Check sheet for the modelled part. Datum: model origin and axes. Units: mm. A direction names the side the tool comes from. Give positions to 0.01 mm unless a question says otherwise; leave off trailing zeros. Order: outer loops, then holes, each group sorted by start corner. A loop starts at its lowest first (then second) coordinate and runs counter-clockwise, first axis right, second up. Notation, with made-up numbers: (69.25, 23) -> (74.25, 23) arc R35 cw to (74.25, 55) -> close; hole circle Ø8 at (0.25, -22.5). An arc over 180 degrees is marked (long way). Answer in a Markdown table with one row per item. Add a question column.
(1) Set-up check for faces 4 (the face through (87, 3, -105)), 5 (the face through (20, 3, -102)), 6 (the face through (55, 3, -20.322)), 7 (the face through (20, 3, -40)): record each of +Z, -Z, +X, -X, +Y, -Y from which the full face is reachable in a straight line by a thin tool's end or side.
(2) Cross-section at A-A (x = 62.5). Record the cut outline in (y, z).
(3) Cross-section at B-B (z = -17). Record the cut outline in (x, y).
(4) Release check for a two-part mould opening along X. For faces 1 (the face through (97, 3, -105)), 2 (the face through (35, 3, -47)), 3 (the face through (29.574, 3.042, -82.14)) record: released by +X, released by -X, zero draft, split by the parting line, or undercut.
(5) Thickness scan on L1, parallel to X at y = 3, z = -48; L2, parallel to X at y = 2.75, z = -44; L3, parallel to X at y = 1.85, z = -17. Record the ranges inside material, lowest first. Write a range as [from, to].
(6) Go/stop test with flat-tipped pins: pin 1 (8.5 mm diameter, centred on x = 70, z = -8, fed in from +Y); pin 2 (2.5 mm diameter, centred on y = 2.5, z = -18.5, fed in from -X); pin 3 (1.4 mm diameter, centred on x = 51.5, y = 2.5, fed in from -Z); pin 4 (3 mm diameter, centred on x = 85, z = -8, fed in from +Y). Record where each tip stops, or that it passes through.
```python
from build123d import *

# Parameters (mm, degrees)
SKETCH1_W           = 100
SKETCH1_H           = 105
BOSS_EXTRUDE1_DEPTH = 6
SKETCH3_W           = 10
SKETCH3_H           = 5
SKETCH3_W_2         = 15
SKETCH3_W_3         = 20
SKETCH3_W_4         = 25
SKETCH3_W_5         = 30
SKETCH3_W_6         = 35
SKETCH3_W_7         = 40
SKETCH3_W_8         = 45
SKETCH3_W_9         = 50
SKETCH3_W_10        = 55
CUT_EXTRUDE1_DEPTH  = 6
SKETCH4_W           = 5
SKETCH4_H           = 80
SKETCH4_H_2         = 75
SKETCH4_H_3         = 70
SKETCH4_H_4         = 65
SKETCH4_H_5         = 60
CUT_EXTRUDE2_DEPTH  = 6
SKETCH5_R           = 1.35
SKETCH5_R_2         = 1.6
SKETCH5_R_3         = 2.1
SKETCH5_R_4         = 2.6
SKETCH5_R_5         = 1.1
SKETCH5_R_6         = 3.1
SKETCH5_R_7         = 3.6
SKETCH5_R_8         = 4.1
CUT_EXTRUDE3_DEPTH  = 7
SKETCH7_W           = 5
SKETCH7_H           = 5
SKETCH7_H_2         = 6
SKETCH7_H_3         = 8
CUT_EXTRUDE4_DEPTH  = 7
CUT_EXTRUDE5_DEPTH  = 7


with BuildPart() as part:
    # Sketch1 → Boss-Extrude1 (new body)
    with BuildSketch(Plane(origin=(0, 0, 0), x_dir=(1, 0, 0), z_dir=(0, 1, 0))):
        with Locations((50, 52.5)):
            Rectangle(SKETCH1_W, SKETCH1_H)
    extrude(amount=BOSS_EXTRUDE1_DEPTH)

    # Sketch3 → Cut-Extrude1 (cut)
    with BuildSketch(Plane(origin=(0, 6, 0), x_dir=(1, 0, 0), z_dir=(0, 1, 0))):
        with Locations((5, 97.5)):
            Rectangle(SKETCH3_W, SKETCH3_H)
        with Locations((7.5, 87.5)):
            Rectangle(SKETCH3_W_2, SKETCH3_H)
        with Locations((10, 77.5)):
            Rectangle(SKETCH3_W_3, SKETCH3_H)
        with Locations((12.5, 67.5)):
            Rectangle(SKETCH3_W_4, SKETCH3_H)
        with Locations((15, 57.5)):
            Rectangle(SKETCH3_W_5, SKETCH3_H)
        with Locations((17.5, 47.5)):
            Rectangle(SKETCH3_W_6, SKETCH3_H)
        with Locations((20, 37.5)):
            Rectangle(SKETCH3_W_7, SKETCH3_H)
        with Locations((22.5, 27.5)):
            Rectangle(SKETCH3_W_8, SKETCH3_H)
        with Locations((25, 17.5)):
            Rectangle(SKETCH3_W_9, SKETCH3_H)
        with Locations((27.5, 7.5)):
            Rectangle(SKETCH3_W_10, SKETCH3_H)
    extrude(amount=-CUT_EXTRUDE1_DEPTH, mode=Mode.SUBTRACT)

    # Sketch4 → Cut-Extrude2 (cut)
    with BuildSketch(Plane(origin=(0, 6, 0), x_dir=(1, 0, 0), z_dir=(0, 1, 0))):
        with Locations((92.5, 65)):
            Rectangle(SKETCH4_W, SKETCH4_H)
        with Locations((82.5, 67.5)):
            Rectangle(SKETCH4_W, SKETCH4_H_2)
        with Locations((72.5, 70)):
            Rectangle(SKETCH4_W, SKETCH4_H_3)
        with Locations((62.5, 72.5)):
            Rectangle(SKETCH4_W, SKETCH4_H_4)
        with Locations((52.5, 75)):
            Rectangle(SKETCH4_W, SKETCH4_H_5)
    extrude(amount=-CUT_EXTRUDE2_DEPTH, mode=Mode.SUBTRACT)

    # Sketch5 → Cut-Extrude3 (cut, through all)
    with BuildSketch(Plane(origin=(0, 6, 0), x_dir=(1, 0, 0), z_dir=(0, 1, 0))):
        with Locations((91, 8)):
            Circle(SKETCH5_R)
        with Locations((85, 8)):
            Circle(SKETCH5_R_2)
        with Locations((78, 8)):
            Circle(SKETCH5_R_3)
        with Locations((70, 8)):
            Circle(SKETCH5_R_4)
        with Locations((96, 8)):
            Circle(SKETCH5_R_5)
        with Locations((90, 17)):
            Circle(SKETCH5_R_6)
        with Locations((80, 17)):
            Circle(SKETCH5_R_7)
        with Locations((69, 17)):
            Circle(SKETCH5_R_8)
    extrude(amount=-CUT_EXTRUDE3_DEPTH, mode=Mode.SUBTRACT)

    # Sketch7 → Cut-Extrude4 (cut, through all)
    with BuildSketch(Plane(origin=(0, 6, 0), x_dir=(1, 0, 0), z_dir=(0, 1, 0))):
        with Locations((22.5, 102.5)):
            Rectangle(SKETCH7_W, SKETCH7_H)
        with Locations((32.5, 102)):
            Rectangle(SKETCH7_W, SKETCH7_H_2)
        with Locations((42.5, 101)):
            Rectangle(SKETCH7_W, SKETCH7_H_3)
    extrude(amount=-CUT_EXTRUDE4_DEPTH, mode=Mode.SUBTRACT)

    # Sketch8 → Cut-Extrude5 (cut, through all)
    with BuildSketch(Plane(origin=(0, 6, 0), x_dir=(1, 0, 0), z_dir=(0, 1, 0))):
        Polygon((65.986104675, 31.416856683), (64.340656408, 34.266856683), (61.049759874, 34.266856683), (59.404311607, 31.416856683), (61.049759874, 28.566856683), (64.340656408, 28.566856683), align=None)
        Polygon((59.309574734, 23.921668245), (57.231113764, 27.521668245), (53.074191826, 27.521668245), (50.995730857, 23.921668245), (53.074191826, 20.321668245), (57.231113764, 20.321668245), align=None)
        Polygon((55.845473118, 34.972078883), (53.478337015, 39.072078883), (48.744064807, 39.072078883), (46.376928704, 34.972078883), (48.744064807, 30.872078883), (53.478337015, 30.872078883), align=None)
        Polygon((46.037567534, 60.151166507), (43.093081161, 65.251166507), (37.204108416, 65.251166507), (34.259622043, 60.151166507), (37.204108416, 55.051166507), (43.093081161, 55.051166507), align=None)
        Polygon((42.884078391, 78.793578101), (39.073566615, 85.393578101), (31.452543062, 85.393578101), (27.642031285, 78.793578101), (31.452543062, 72.193578101), (39.073566615, 72.193578101), align=None)
    extrude(amount=-CUT_EXTRUDE5_DEPTH, mode=Mode.SUBTRACT)


solid = part.part
```
Answer below:
| question | item | result |
|---|---|---|
| 1 | face 4 | -Z, +X, -X, +Y, -Y |
| 1 | face 5 | -Z, +Y, -Y |
| 1 | face 6 | +Y, -Y |
| 1 | face 7 | -X, +Y, -Y |
| 2 | outline | (0, -40) -> (6, -40) -> (6, -34.27) -> (0, -34.27) -> close; (0, -28.57) -> (6, -28.57) -> (6, 0) -> (0, 0) -> close |
| 3 | outline | (50, 0) -> (64.9, 0) -> (64.9, 6) -> (50, 6) -> close; (73.1, 0) -> (76.4, 0) -> (76.4, 6) -> (73.1, 6) -> close; (83.6, 0) -> (86.9, 0) -> (86.9, 6) -> (83.6, 6) -> close; (93.1, 0) -> (100, 0) -> (100, 6) -> (93.1, 6) -> close |
| 4 | face 1 | zero draft |
| 4 | face 2 | released by -X |
| 4 | face 3 | undercut |
| 5 | L1 | x = [35, 50], [55, 60], [65, 70], [75, 80], [85, 90], [95, 100] |
| 5 | L2 | x = [0, 60], [65, 70], [75, 80], [85, 90], [95, 100] |
| 5 | L3 | x = [50, 64.9], [73.1, 76.4], [83.6, 86.9], [93.1, 100] |
| 6 | pin 1 | stops at y = 6 |
| 6 | pin 2 | stops at x = 50 |
| 6 | pin 3 | stops at z = -45 |
| 6 | pin 4 | passes through |
